```python
from build123d import *

# Parameters (mm, degrees)
SKETCH1_W           = 15
SKETCH1_H           = 29
BOSS_EXTRUDE1_DEPTH = 147
SKETCH2_R           = 3.2
CUT_EXTRUDE1_DEPTH  = 9.5


with BuildPart() as part:
    # Sketch1 → Boss-Extrude1 (new body)
    with BuildSketch(Plane.XY):
        with Locations((-34.484924623, 20.173366834)):
            Rectangle(SKETCH1_W, SKETCH1_H)
    extrude(amount=BOSS_EXTRUDE1_DEPTH)

    # Sketch2 → Cut-Extrude1 (cut)
    with BuildSketch(Plane.XY.offset(147)):
        with Locations((-34.484924623, 20.173366834)):
            Circle(SKETCH2_R)
    cut_extrude1 = extrude(amount=-CUT_EXTRUDE1_DEPTH, mode=Mode.SUBTRACT)

    # Mirror1: Cut-Extrude1 across plane
    add(cut_extrude1.mirror(Plane.XY.offset(73.5)), mode=Mode.SUBTRACT)


solid = part.part
```
Geometry check sheet. Reference: the model listing, model coordinates, mm. A direction names the side the tool comes from. Give positions to 0.01 mm unless a question says otherwise; leave off trailing zeros. Order: outer loops, then holes, each group sorted by start corner. A loop starts at its lowest first (then second) coordinate and runs counter-clockwise, first axis right, second up.
1. Thickness scan on L1, parallel to Y at x = -32.5, z = 138.5; L2, parallel to Z at x = -34.25, y = 22.5. Record the ranges inside material, lowest first.
2. Release check for a two-part mould opening along Y. For faces 4 (the face through (-35, 34.673, 72)), 5 (the face through (-41.985, 20, 72)), 6 (the face through (-37.682, 20.314, 142.316)), 7 (the face through (-35, 5.673, 72)) record: pulls with the +Y half, pulls with the -Y half, needs draft (parallel to the pull), parting line crosses it, or undercut.
3. Access from +Z, -Z, +X, -X, +Y, -Y to the whole of each face (thin tool, end or side, straight path). Record for faces 1 (the face through (-35, 20, 137.5)), 2 (the face through (-37.682, 20.314, 4.684)), 3 (the face through (-35, 24, 147)).
4. Gauge pin test, flat ends, axial feed: pin 1 Ø3 at (x, y) = (-36, 18.5) entering from +Z; pin 2 Ø5 at (x, y) = (-34.48, 20.17) entering from +Z. Record the tip position at first contact, or that the pin passes through.
5. Section check A-A, the plane x = -32.75. Enter the section's corners in (y, z), and give its area (3 significant figures).
Values follow:
1. L1: y = 5.67 to 17.66, 22.68 to 34.67
1. L2: z = 9.5 to 137.5
2. face 4: pulls with the +Y half
2. face 5: needs draft
2. face 6: undercut
2. face 7: pulls with the -Y half
3. face 1: +Z
3. face 2: -Z
3. face 3: +Z, +X, -X, +Y, -Y
4. pin 1: stops at z = 147
4. pin 2: stops at z = 137.5
5. outline: (5.67, 0) - (17.48, 0) - (17.48, 9.5) - (22.86, 9.5) - (22.86, 0) - (34.67, 0) - (34.67, 147) - (22.86, 147) - (22.86, 137.5) - (17.48, 137.5) - (17.48, 147) - (5.67, 147) - close
5. area: 4,160 mm2
